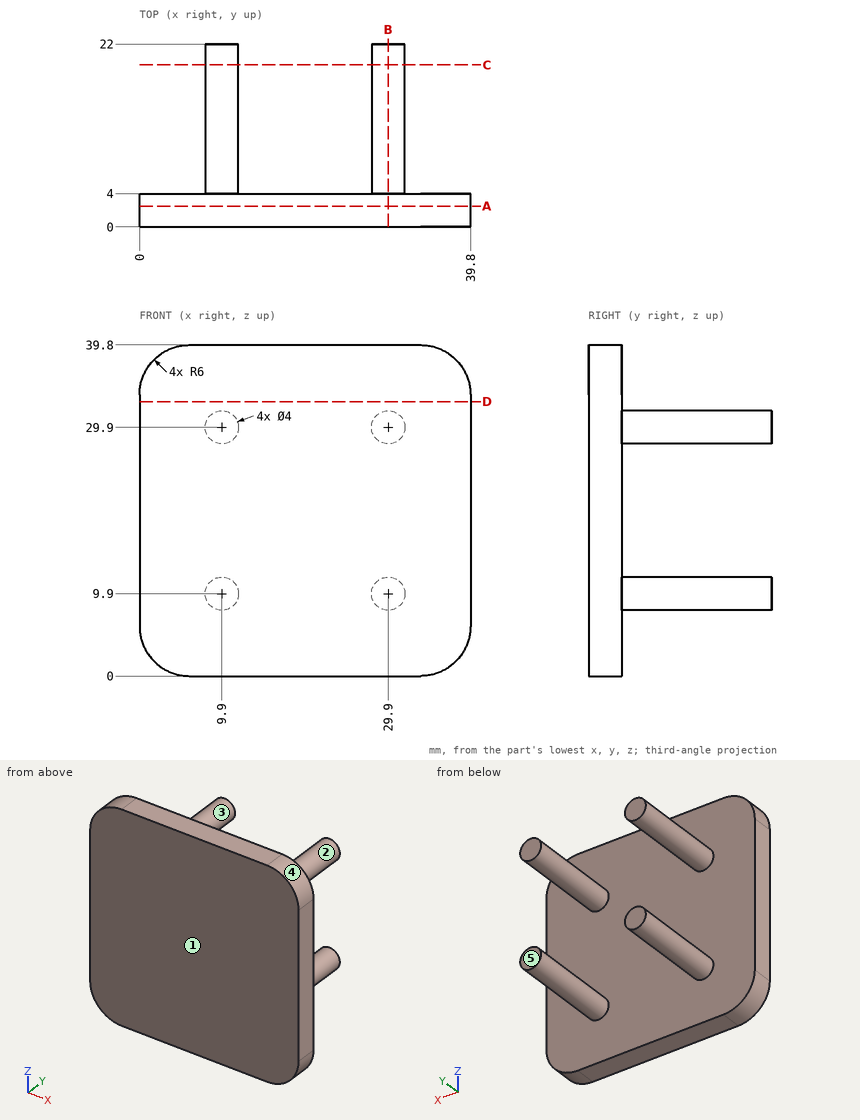
For this review, use the dimensioned drawing (mm, ordinates from the lowest corner) and the shaded views. A direction names the side the tool comes from. Give positions to 0.01 mm unless a question says otherwise; leave off trailing zeros. Order: outer loops, then holes, each group sorted by start corner. A loop starts at its lowest first (then second) coordinate and runs counter-clockwise, first axis right, second up. Notation, with made-up numbers: M -26.75,2 L 18.25,2 A17 cw 18.25,16 Z; hole C 40,31.25 d10. An arc over 180 degrees is marked long. One line per question, with ' | ' between items. Start each with the question number.
1) Clearance check with flat-ended pins moving along their axes: P1, Ø10, axis at x = 21, z = 22, coming from the +Y side; P2, Ø3, axis at x = 13, y = 19.5, coming from the +Z side; P3, Ø8, axis at y = 13.5, z = 11, coming from the -X side. State where each tip first meets the part, or that it passes through.
2) Consider section D-D, the plane z = 33. Give the boundary of the cut face in (x, y).
3) For the marked faces 1 and 2, list the 3-axis set-ups (+Z, -Z, +X, -X, +Y, -Y) from which the entire face can be reached by the end or side of a thin tool; tool diameter is ignored.
4) Wall thickness on L1, parallel to Y at x = 32, z = 20; L2, parallel to X at y = 9.75, z = 10.5; L3, parallel to X at y = 21.25, z = 9: over which ranges is each line inside the solid? List them lowest first. Write a range as from..to.
5) Consider section A-A, the plane y = 2.5. Give the boundary of the cut face in (x, z), then the cut area to 3 significant figures.
6) Consider section B-B, the plane x = 29.9. Give the boundary of the cut face in (y, z), then the cut area to 3 significant figures.
7) Mouldability with a two-part tool opening along Z and no side actions: class the marked faces 3, 4 and 5 as pulls with the +Z half, pulls with the -Z half, needs draft (parallel to the pull), parting line crosses it, or undercut.
8) Consider section C-C, the plane y = 19.5. Give the boundary of the cut face in (x, z).
Found:
1) P1: stops at y = 4 | P2: stops at z = 31.1 | P3: stops at x = 7.9
2) outline: M 0,0 L 39.8,0 L 39.8,4 L 0,4 Z
3) face 1: +Z, -Z, +X, -X, -Y | face 2: +Y
4) L1: y = 0..4 | L2: x = 7.99..11.81, 27.99..31.81 | L3: x = 8.11..11.69, 28.11..31.69
5) outline: M 0,6 A6 ccw 6,0 L 33.8,0 A6 ccw 39.8,6 L 39.8,33.8 A6 ccw 33.8,39.8 L 6,39.8 A6 ccw 0,33.8 Z | area: 1,550 mm²
6) outline: M 0,0 L 4,0 L 4,7.9 L 22,7.9 L 22,11.9 L 4,11.9 L 4,27.9 L 22,27.9 L 22,31.9 L 4,31.9 L 4,39.8 L 0,39.8 Z | area: 303 mm²
7) face 3: undercut | face 4: pulls with the +Z half | face 5: needs draft
8) outline: C 9.9,9.9 d4; C 9.9,29.9 d4; C 29.9,9.9 d4; C 29.9,29.9 d4
